```python
from build123d import *

# Parameters (mm, degrees)
F0_R     = 6.858
F1_DEPTH = 4.7625


with BuildPart() as f1:
    # F0 (on Top) → F1 (new body)
    with BuildSketch(Plane.XY):
        with BuildLine():
            ThreePointArc((-33.360649, 13.814234), (-34.603048, 0.046057), (-33.376957, -13.723581))
            ThreePointArc((-33.376957, -13.723581), (-29.549678, -23.21519), (-22.156792, -30.292191))
            Line((-22.156792, -30.292191), (11.323438, -51.212653))
            ThreePointArc((11.323438, -51.212653), (42.490556, -60.360838), (73.897804, -52.074505))
            Line((73.897804, -52.074505), (108.839764, -30.261436))
            ThreePointArc((108.839764, -30.261436), (116.142274, -23.23358), (119.984489, -13.855157))
            ThreePointArc((119.984489, -13.855157), (121.301479, -0.00415), (119.985359, 13.84694))
            ThreePointArc((119.985359, 13.84694), (116.14346, 23.236597), (108.83063, 30.26855))
            Line((108.83063, 30.26855), (75.312555, 51.212004))
            ThreePointArc((75.312555, 51.212004), (43.309839, 60.395046), (11.308, 51.208947))
            Line((11.308, 51.208947), (-22.223896, 30.269336))
            ThreePointArc((-22.223896, 30.269336), (-29.510199, 23.204472), (-33.360649, 13.814234))
        make_face()
        with Locations((-9.860053, 0)):
            Circle(F0_R, mode=Mode.SUBTRACT)
        with BuildLine():
            ThreePointArc((87.726747, 0), (43.302147, -44.4246), (-1.122453, 0))
            ThreePointArc((-1.122453, 0), (43.302147, 44.4246), (87.726747, 0))
        make_face(mode=Mode.SUBTRACT)
        with BuildLine():
            ThreePointArc((103.347747, 0), (96.489747, -6.858), (89.631747, 0))
            ThreePointArc((89.631747, 0), (96.489747, 6.858), (103.347747, 0))
        make_face(mode=Mode.SUBTRACT)
    extrude(amount=F1_DEPTH)


solid = f1.part
```
For this review, take the finished solid that the model builds, in its own axes (mm). Coordinates: 2 decimals unless noted, no trailing zeros. Write each loop counter-clockwise with the first axis right and the second up, starting at its lowest first coordinate (ties: lowest second). Pieces come first, ordered by that corner, then holes. Notation, with made-up numbers: (-18, 64.25) - (30, 64.25) arc R30 ccw to (30, 88.25) - close; hole circle Ø11 at (11.25, 81). An arc over 180 degrees is marked (long way). Put each result on its own line as item: value.
1. Wall thickness on probe 1 along Y at (x, z) = (44.5, 1.9); probe 2 along Y at (x, z) = (95, 2.8); probe 3 along X at (y, z) = (16, 3.8): over which ranges is each line inside the solid? List them lowest first.
Values found:
probe 1: -60.36 to -44.41, 44.41 to 60.38
probe 2: -38.9 to -6.69, 6.69 to 38.91
probe 3: -32.85 to 1.86, 84.75 to 119.49
2. Add section D-D, the plane x = 2. Give the boundary of the cut face in (y, z), then the cut area to 3 significant figures.
Values found:
outline: (-45.39, 0) - (-16.36, 0) - (-16.36, 4.76) - (-45.39, 4.76) - close; (16.36, 0) - (45.4, 0) - (45.4, 4.76) - (16.36, 4.76) - close
area: 277 mm²
3. For pin 1 (11 mm diameter, centred on x = -9.86, y = 0, fed in from +Z); pin 2 (1 mm diameter, centred on y = -10, z = 1, fed in from -X), all flat-tipped, find the tip position at first contact; note any pin that passes through.
Values found:
pin 1: through
pin 2: x = -34.02
4. Add section A-A, the plane y = 0. Give the boundary of the cut face in (x, z), then the cut area to 3 significant figures.
Values found:
outline: (-34.6, 0) - (-16.72, 0) - (-16.72, 4.76) - (-34.6, 4.76) - close; (-3, 0) - (-1.12, 0) - (-1.12, 4.76) - (-3, 4.76) - close; (87.73, 0) - (89.63, 0) - (89.63, 4.76) - (87.73, 4.76) - close; (103.35, 0) - (121.3, 0) - (121.3, 4.76) - (103.35, 4.76) - close
area: 189 mm²
5. Add section C-C, the plane y = 41.5. Give the boundary of the cut face in (x, z), then the cut area to 3 significant figures.
Values found:
outline: (-4.24, 0) - (27.45, 0) - (27.45, 4.76) - (-4.24, 4.76) - close; (59.15, 0) - (90.86, 0) - (90.86, 4.76) - (59.15, 4.76) - close
area: 302 mm²
6. Mouldability with a two-part tool opening along X and no side actions: class faces 1 (the cylindrical face through (103.34, 0.3, 2.35)), 2 (the flat face through (-5.2, 40.9, 2.3)), 3 (the flat face through (89, 0, 4.762)) as released by +X, released by -X, zero draft, split by the parting line, or undercut.
Values found:
face 1: undercut
face 2: released by -X
face 3: zero draft
7. Add section B-B, the plane z = 3.4. Give the boundary of the cut face in (x, y) (1 decimal), then the cut area to 3 significant figures.
Values found:
outline: (-33.4, -13.7) arc R24.3 ccw to (-22.2, -30.3) - (11.3, -51.2) arc R60.5 ccw to (73.9, -52.1) - (108.8, -30.3) arc R24.6 ccw to (120, -13.9) arc R73.5 ccw to (120, 13.8) arc R24.5 ccw to (108.8, 30.3) - (75.3, 51.2) arc R60.3 ccw to (11.3, 51.2) - (-22.2, 30.3) arc R24.8 ccw to (-33.4, 13.8) arc R77.4 ccw to start; hole circle Ø13.7 at (-9.9, 0); hole circle Ø88.8 at (43.3, 0); hole circle Ø13.7 at (96.5, 0)
area: 7,460 mm²
